from build123d import *

# Parameters (mm, degrees)
PER_AGE1_D = 6.6


with BuildPart() as part:
    # Esquisse1 → Base-Révolution (revolve)
    with BuildSketch(Plane.XY, mode=Mode.PRIVATE) as base_r_volution_sk:
        Polygon((0, 22.5), (0, 30), (3, 30), (3, 47.5), (13, 47.5), (13, 29), (110, 29), (110, 21), (98, 21), (98, 19), (32, 19), (32, 21), (20, 21), (20, 22.5), align=None)
    revolve(base_r_volution_sk.sketch.rotate(Axis((-23.254623921, 0, 0), (1, 0, 0)), 90), axis=Axis((-23.254623921, 0, 0), (1, 0, 0)))

    # Perçage1 (through all)
    with Locations(Plane.ZY.offset(-3)):
        with Locations((0, 40), (40, 0), (-40, 0), (0, -40)):
            Hole(PER_AGE1_D / 2)


solid = part.part
Could you check a few things on this model? Use its own coordinates, in mm. A direction names the side the tool comes from. Give positions to 0.01 mm unless a question says otherwise; leave off trailing zeros. Order: outer loops, then holes, each group sorted by start corner. A loop starts at its lowest first (then second) coordinate and runs counter-clockwise, first axis right, second up.
1. Suppose I cut it at A-A (y = 5). Write out the boundary of the cut face in (x, z).
Answers below:
outline: (0, -29.58) - (3, -29.58) - (3, -47.24) - (13, -47.24) - (13, -28.57) - (110, -28.57) - (110, -20.4) - (98, -20.4) - (98, -18.33) - (32, -18.33) - (32, -20.4) - (20, -20.4) - (20, -21.94) - (0, -21.94) - close; (0, 21.94) - (20, 21.94) - (20, 20.4) - (32, 20.4) - (32, 18.33) - (98, 18.33) - (98, 20.4) - (110, 20.4) - (110, 28.57) - (13, 28.57) - (13, 47.24) - (3, 47.24) - (3, 29.58) - (0, 29.58) - close
2. Suppose I cut it at C-C (z = -40). Write out the boundary of the cut face in (x, y), plus the area to 3 significant figures.
Answers below:
outline: (3, -25.62) - (13, -25.62) - (13, -3.3) - (3, -3.3) - close; (3, 3.3) - (13, 3.3) - (13, 25.62) - (3, 25.62) - close
area: 446 mm2
3. Which directions (+Z, -Z, +X, -X, +Y, -Y) give clear straight access to the entire face, cutting with the end or side of a thin tool? Please do faces 1 (the cylindrical face through (8.07, -2.008, 42.619)), 2 (the cylindrical face through (103.92, -6.31, 20.03)), 3 (the flat face through (32, 11, 16)).
Answers below:
face 1: +X, -X
face 2: +X
face 3: -X
4. Suppose I cut it at D-D (y = 24.5). Write out the boundary of the cut face in (x, z).
Answers below:
outline: (0, -17.31) - (3, -17.31) - (3, -40.69) - (13, -40.69) - (13, -15.52) - (110, -15.52) - (110, 15.52) - (13, 15.52) - (13, 40.69) - (3, 40.69) - (3, 17.31) - (0, 17.31) - close
5. I need wall thicknesses on L1, parallel to Y at x = 7.75, z = 0; L2, parallel to Y at x = 102.25, z = 0; L3, parallel to Z at x = 8.5, y = 2. Which ranges of each line are inside material? Lowest first, please.
Answers below:
L1: y = -47.5 to -43.3, -36.7 to -22.5, 22.5 to 36.7, 43.3 to 47.5
L2: y = -29 to -21, 21 to 29
L3: z = -47.46 to -42.62, -37.38 to -22.41, 22.41 to 37.38, 42.62 to 47.46
6. Suppose I cut it at B-B (x = 25.5). Write out the boundary of the cut face in (y, z), plus the area to 3 significant figures.
Answers below:
outline: circle Ø58 at (0, 0); hole circle Ø42 at (0, 0)
area: 1,260 mm2
7. For pin 1 (4 mm diameter, centred on x = 35, z = -27, fed in from -Y); pin 2 (8 mm diameter, centred on x = 95.5, z = -10.5, fed in from +Y); pin 3 (2 mm diameter, centred on x = 42.5, z = 21.5, fed in from +Y), each with a flat end and sliding along its axis, tell me the tip position at first contact or that it passes through.
Answers below:
pin 1: stops at y = -14.7
pin 2: stops at y = 28.26
pin 3: stops at y = 20.51
8. Thinking about a two-plate mould opening in Y: for faces 4 (the flat face through (98, 11, -16)), 5 (the cylindrical face through (1.521, -25.296, 16.128)), 6 (the flat face through (13, -22, 20)), which applies, +Y half, -Y half, draft (parallel to the pull), parting line (faces both ways), or undercut?
Answers below:
face 4: undercut
face 5: parting line
face 6: draft
